```python
from build123d import *

# Parameters (mm, degrees)
SKETCH1_W               = 28.4
SKETCH1_H               = 28.4
BOSS_EXTRUDE1_DEPTH     = 2
SKETCH1_3_W             = 28.4
SKETCH1_3_H             = 28.4
BOSS_EXTRUDE2_DEPTH     = 11.52
M2_5_TAPPED_HOLE1_D     = 2.05
M2_5_TAPPED_HOLE1_DEPTH = 6.35
M2_5_TAPPED_HOLE1_TIP   = 0.615882135


with BuildPart() as part:
    # Sketch1 → Boss-Extrude1 (new body)
    with BuildSketch(Plane(origin=(0, 0, 0), x_dir=(1, 0, 0), z_dir=(0, 1, 0))):
        Rectangle(SKETCH1_W, SKETCH1_H)
        Polygon((-14.2, 14.2), (-20.5, 0), (-14.2, -14.2), align=None)
        Polygon((20.5, 0), (14.2, -14.2), (14.2, 14.2), align=None)
    extrude(amount=BOSS_EXTRUDE1_DEPTH)

    # Sketch1_3 → Boss-Extrude2 (add)
    with BuildSketch(Plane(origin=(0, 0, 0), x_dir=(1, 0, 0), z_dir=(0, 1, 0))):
        Rectangle(SKETCH1_3_W, SKETCH1_3_H)
    extrude(amount=BOSS_EXTRUDE2_DEPTH)

    # M2.5 Tapped Hole1
    with Locations(Plane(origin=(0, 2, 0), x_dir=(1, 0, 0), z_dir=(0, 1, 0))):
        with Locations((-17.5, 0), (17.5, 0)):
            Hole(M2_5_TAPPED_HOLE1_D / 2, depth=M2_5_TAPPED_HOLE1_DEPTH)
            with Locations((0, 0, -(M2_5_TAPPED_HOLE1_DEPTH + M2_5_TAPPED_HOLE1_TIP / 2))):  # 118° drill point
                Cone(0, M2_5_TAPPED_HOLE1_D / 2, M2_5_TAPPED_HOLE1_TIP, mode=Mode.SUBTRACT)


solid = part.part
```
CAD build for the part. Positions are in the model's coordinates, mm. A direction names the side the tool comes from. Coordinates: 2 decimals unless noted, no trailing zeros. Order: outer loops, then holes, each group sorted by start corner. A loop starts at its lowest first (then second) coordinate and runs counter-clockwise, first axis right, second up. Notation, with made-up numbers: M 57.25,35 L 83.25,35 A8 ccw 83.25,42 Z; hole C 80.5,-38.5 d4. An arc over 180 degrees is marked long. Write each question's results on one line, items separated by ' | '. Start each with the question number.
Q1. Flat gauge pins, fed straight in: P1, Ø5, axis at y = 5.5, z = 2.5, coming from the +X side; P2, Ø3, axis at x = 18, z = 1.5, coming from the +Y side; P3, Ø1.6, axis at x = 17.5, z = 0, coming from the +Y side; P4, Ø3, axis at y = 4.5, z = -4, coming from the -X side. Where does each tip first touch, or does it go through?
Q2. Which spindle directions (+Z, -Z, +X, -X, +Y, -Y) get a long thin tool onto all of the face, cutting with end or side? Do faces 1 (the flat face through (-14.2, 7, 0)), 2 (the flat face through (0, 6, -14.2)), 3 (the flat face through (16, 2, 0)). Say none if no direction does.
Q3. Drill centre lines: probe 1 along X at (y, z) = (4, -7); probe 2 along Z at (x, y) = (-17.5, 0.7) (3 decimals); probe 3 along Y at (x, z) = (-15, 5.25). Where is each one in solid material? Low to high. Write a range as from..to.
Q4. Pull direction Z, two halves, no side cores. Call faces 4 (the cylindrical face through (-16.476, 0.986, -0.045)), 5 (the flat face through (0, 11.52, 0)), 6 (the flat face through (17.306, 0.986, -7.199)): +Z half, -Z half, draft (parallel to the pull), parting line (faces both ways), or undercut.
Q5. Cut at B-B (z = -10.5). List the corners of the cut face in (x, y).
Q6. Cut at D-D (z = 11.5). List the corners of the cut face in (x, y), then the cut area to 3 significant figures.
Q7. Cut at A-A (x = 17.5). List the corners of the cut face in (y, z) (3 decimals), then the cut area to 3 significant figures.
Q8. Cut at C-C (y = 4). List the corners of the cut face in (x, z).
Found:
1) P1: x = 14.2 | P2: y = 2 | P3: through | P4: x = -14.2
2) face 1: +Z, -Z, -X, +Y | face 2: -Z, +X, -X, +Y, -Y | face 3: +Z, -Z, +X, +Y
3) probe 1: -14.2..14.2 | probe 2: -6.762..-1.025, 1.025..6.762 | probe 3: 0..2
4) face 4: undercut | face 5: draft | face 6: -Z half
5) outline: M -15.84,0 L 15.84,0 L 15.84,2 L 14.2,2 L 14.2,11.52 L -14.2,11.52 L -14.2,2 L -15.84,2 Z
6) outline: M -15.4,0 L 15.4,0 L 15.4,2 L 14.2,2 L 14.2,11.52 L -14.2,11.52 L -14.2,2 L -15.4,2 Z | area: 332 mm²
7) outline: M 0,-6.762 L 2,-6.762 L 2,-1.025 L 0,-1.025 Z; M 0,1.025 L 2,1.025 L 2,6.762 L 0,6.762 Z | area: 22.9 mm²
8) outline: M -14.2,-14.2 L 14.2,-14.2 L 14.2,14.2 L -14.2,14.2 Z
